Part model, mm, in its own coordinate system. Face numbers are marked on the shaded views. Give positions to 0.01 mm unless a question says otherwise; leave off trailing zeros. Write each loop counter-clockwise with the first axis right and the second up, starting at its lowest first coordinate (ties: lowest second). Pieces come first, ordered by that corner, then holes. Notation, with made-up numbers: (-35, 53) - (17, 53) arc R22 ccw to (17, 90) - close; hole circle Ø8 at (37.25, 81.25). An arc over 180 degrees is marked (long way). Answer in a Markdown table with one row per item. Add a question column.
1. Pull direction Y, two halves, no side cores. Call the marked faces 1, 2, 3 and 4: released by +Y, released by -Y, zero draft, split by the parting line, or undercut.
2. Band-saw the part on B-B on y = 0. Write the cut outline in (x, z), plus the area to 3 significant figures.
3. Probe line 1 along Y through (x, z) = (-0.7, -6); line 2 along Z through (x, y) = (-0.5, -0.25); line 3 along Y through (x, z) = (0.5, 6.5). List the from-to ranges inside material, lowest first.
4. Band-saw the part on A-A on z = -0.25. Write the cut outline in (x, y), plus the area to 3 significant figures.
5. Drop flat-ended pins along their axis: pin 1 Ø2.5 at (x, y) = (0, 0) entering from +Z; pin 2 Ø1.5 at (x, z) = (-1, -2) entering from -Y. Give the stop position or say it passes through.
6. Band-saw the part on D-D on x = -1.1. Write the cut outline in (y, z), plus the area to 3 significant figures.
7. Band-saw the part on C-C on z = -6. Write the cut outline in (x, y).
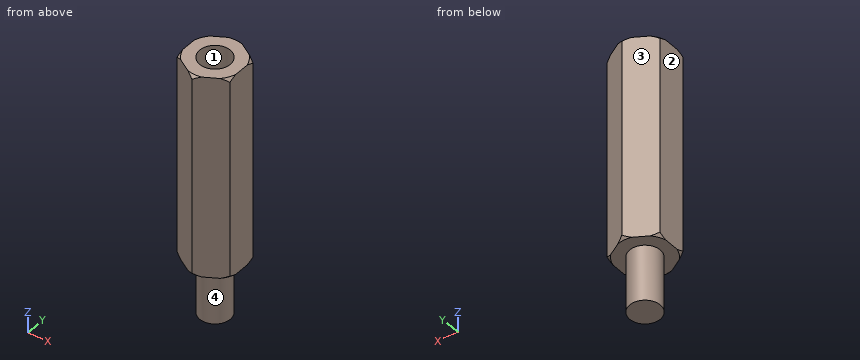
```python
from build123d import *

# Parameters (mm, degrees)
PAD_DEPTH    = 10
SKETCH001_R  = 1.5
POCKET_DEPTH = 15
SKETCH002_R  = 1.5
PAD001_DEPTH = 5.5


with BuildPart() as body001:
    # Sketch003 → Revolution (revolve)
    with BuildSketch(Plane.YZ):
        Polygon((2.2, 10.5), (5.2, 10.5), (5.2, -10.5), (2.2, -10.5), (3.444538, -9.255462), (3.444538, 9.255462), align=None)
    revolve(axis=Axis((0, 0, 0), (0, 0, 1)))


with BuildPart() as cut:
    # Sketch → Pad (new body, symmetric)
    with BuildSketch(Plane.XY):
        Polygon((2.6, 1.501111), (0, 3.002221), (-2.6, 1.501111), (-2.6, -1.501111), (0, -3.002221), (2.6, -1.501111), align=None)
    extrude(amount=PAD_DEPTH, both=True)

    # Sketch001 (on Face8 of Pad) → Pocket (cut)
    with BuildSketch(Plane.XY.offset(10)):
        Circle(SKETCH001_R)
    extrude(amount=-POCKET_DEPTH, mode=Mode.SUBTRACT)

    # Sketch002 (on Face4 of Pocket) → Pad001 (join)
    with BuildSketch(Plane(origin=(0, 0, -10), x_dir=(1, 0, 0), z_dir=(0, 0, -1))):
        Circle(SKETCH002_R)
    extrude(amount=PAD001_DEPTH)

    # Cut: cut Body001
    add(body001.part, mode=Mode.SUBTRACT)


solid = cut.part
```
Values:
| question | item | result |
|---|---|---|
| 1 | face 1 | undercut |
| 1 | face 2 | zero draft |
| 1 | face 3 | released by +Y |
| 1 | face 4 | split by the parting line |
| 2 | outline | (-2.6, -10) - (-1.5, -10) - (-1.5, -15.5) - (1.5, -15.5) - (1.5, -10) - (2.6, -10) - (2.6, 10) - (1.5, 10) - (1.5, -5) - (-1.5, -5) - (-1.5, 10) - (-2.6, 10) - close |
| 2 | area | 75.5 mm² |
| 3 | line 1 | y = -2.6 to 2.6 |
| 3 | line 2 | z = -15.5 to -5 |
| 3 | line 3 | y = -2.71 to -1.41, 1.41 to 2.71 |
| 4 | outline | (-2.6, -1.5) - (0, -3) - (2.6, -1.5) - (2.6, 1.5) - (0, 3) - (-2.6, 1.5) - close; hole circle Ø3 at (0, 0) |
| 4 | area | 16.3 mm² |
| 5 | pin 1 | stops at z = -5 |
| 5 | pin 2 | stops at y = -2.86 |
| 6 | outline | (-2.37, -10) - (-1.02, -10) - (-1.02, -15.5) - (1.02, -15.5) - (1.02, -10) - (2.37, -10) - (2.37, 10) - (1.02, 10) - (1.02, -5) - (-1.02, -5) - (-1.02, 10) - (-2.37, 10) - close |
| 6 | area | 75.3 mm² |
| 7 | outline | (-2.6, -1.5) - (0, -3) - (2.6, -1.5) - (2.6, 1.5) - (0, 3) - (-2.6, 1.5) - close |
